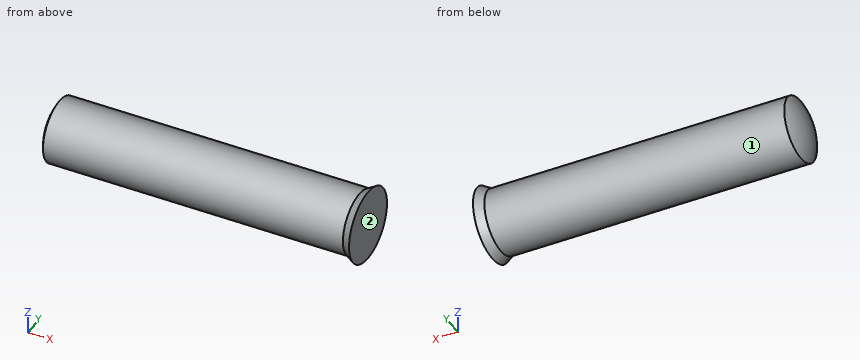
from build123d import *

# Parameters (mm, degrees)
F0_R     = 1.9939
F1_DEPTH = 19.9644


with BuildPart() as f1:
    # F0 (on Right) → F1 (new body)
    with BuildSketch(Plane.YZ):
        Circle(F0_R)
    extrude(amount=-F1_DEPTH)

    # F2 (on Top) → F3 (revolve)
    with BuildSketch(Plane.XY):
        Polygon((-0.549926, 1.9939), (-0.594271, 1.9939), (-0.594271, 0), (0, 0), (0, 1.9939), (0, 2.3114), align=None)
    revolve(axis=Axis((-0.297135, 0, 0), (-1, 0, 0)))

    # F4 (on Top) → F5 (revolve, cut)
    with BuildSketch(Plane.XY):
        with BuildLine():
            Line((-19.939, 0), (-19.9644, 0))
            Line((-19.9644, 0), (-19.9644, -1.9939))
            Line((-19.9644, -1.9939), (-19.416251, -1.9939))
            ThreePointArc((-19.416251, -1.9939), (-19.806141, -1.030643), (-19.939, 0))
        make_face()
    revolve(axis=Axis((-19.9517, 0, 0), (1, 0, 0)), mode=Mode.SUBTRACT)


solid = f1.part
Geometry: final body of the model. Coordinates: model frame, mm. Face numbers are marked on the shaded views. A direction names the side the tool comes from. Round coordinates to 2 decimals unless told otherwise and drop trailing zeros. Order: outer loops, then holes, each group sorted by start corner. A loop starts at its lowest first (then second) coordinate and runs counter-clockwise, first axis right, second up.
Q1. Section A-A, the plane x = -5.75. Output: boundary loops of the cut face in (y, z), and give its area (3 significant figures).
Result sheet:
outline: circle Ø3.99 at (0, 0)
area: 12.5 mm2
Q2. Pin query (flat end, axial travel): pin 1 (1 mm diameter, centred on y = 0.5, z = -0.5, fed in from -X). Return the tip coordinate at first contact, or that it passes through.
Result sheet:
pin 1: stops at x = -19.93
Q3. Access query for the marked faces 1 and 2. Directions: +Z, -Z, +X, -X, +Y, -Y. A direction counts if a zero-diameter tool reaches every point of the face in a straight line with its end or side. Return the directions, or none.
Result sheet:
face 1: -X
face 2: +Z, -Z, +X, +Y, -Y
Q4. Material intervals for probe 1 along Z at (x, y) = (-4.25, -0.1); probe 2 along Y at (x, z) = (-19, -0.9), sorted ascending.
Result sheet:
probe 1: z = -1.99 to 1.99
probe 2: y = -1.78 to 1.78
